Autodesk Inventor part; units mm, degrees
ref_plane "YZ Plane" through (0, 0, 0) normal (1, 0, 0) x (0, 1, 0)
ref_plane "XZ Plane" through (0, 0, 0) normal (0, 1, 0) x (-1, 0, 0)
ref_plane "XY Plane" through (0, 0, 0) normal (0, 0, 1) x (1, 0, 0)
sketch "Skizze1" plane through (0, 0, 0) normal (0, 1, 0) x (-1, 0, 0)
  line L0 (0, 0) -> (-79.5, 0)
  line L1 (-79.5, 0) -> (-79.5, -51.5)
  line L2 (-79.5, -51.5) -> (0, -51.5)
  line L3 (0, -51.5) -> (0, 0)
  line L4 (-30.25, -15.25) -> (-49.25, -15.25)
  line L5 (-49.25, -15.25) -> (-49.25, -36.25)
  line L6 (-49.25, -36.25) -> (-30.25, -36.25)
  line L7 (-30.25, -36.25) -> (-30.25, -15.25)
  point P0 (-39.75, -36.25)
  point P1 (-39.75, -51.5)
  point P2 (-49.25, -25.75)
  point P3 (-79.5, -25.75)
  dimension "d0" = 79.5
  dimension "d1" = 51.5
  dimension "d4" = 21
  dimension "d5" = 19
extrude "Extrusion1" add sketch "Skizze1" along normal blind 3
properties part number "wood_front"
CAD build for the part. Positions are in the model's coordinates, mm. A direction names the side the tool comes from. Round coordinates to 2 decimals unless told otherwise and drop trailing zeros. Order: outer loops, then holes, each group sorted by start corner. A loop starts at its lowest first (then second) coordinate and runs counter-clockwise, first axis right, second up. Notation, with made-up numbers: (34.25, -27.5) -> (53.25, -27.5) arc R19 ccw to (53.25, -9.5) -> close; hole circle Ø2 at (-24, 20.5). An arc over 180 degrees is marked (long way). Write item = value, one per line. Start each with the question number.
(1) Cut at B-B, the plane x = 33. List the corners of the cut face in (y, z), then the cut area to 3 significant figures.
(2) Which spindle directions (+Z, -Z, +X, -X, +Y, -Y) get a long thin tool onto all of the face, cutting with end or side? Do faces 1 (the flat face through (40, 1, -51.5)), 2 (the flat face through (49.25, 1, -26)). Say none if no direction does.
(3) Cut at A-A, the plane z = -35. List the corners of the cut face in (x, y), then the cut area to 4 significant figures.
(4) Cut at C-C, the plane y = 1.3. List the corners of the cut face in (x, z), then the cut area to 3 significant figures.
(5) Probe line 1 (Z direction, x = 41, y = 1.15); line 2 (X direction, y = 0.8, z = -22.5). List the from-to ranges inside material, lowest first. Write a range as [from, to].
(6) Pull direction X, two halves, no side cores. Call faces 3 (the flat face through (79.5, 1, -25)), 4 (the flat face through (40, 0, -14)), 5 (the flat face through (30.25, 1, -26)): released by +X, released by -X, zero draft, split by the parting line, or undercut.
Model answer:
q1.outline = (0, -51.5) -> (3, -51.5) -> (3, -36.25) -> (0, -36.25) -> close; (0, -15.25) -> (3, -15.25) -> (3, 0) -> (0, 0) -> close
q1.area = 91.5 mm2
q2.face_1 = -Z, +X, -X, +Y, -Y
q2.face_2 = +Y, -Y
q3.outline = (0, 0) -> (30.25, 0) -> (30.25, 3) -> (0, 3) -> close; (49.25, 0) -> (79.5, 0) -> (79.5, 3) -> (49.25, 3) -> close
q3.area = 181.5 mm2
q4.outline = (0, -51.5) -> (79.5, -51.5) -> (79.5, 0) -> (0, 0) -> close; hole (30.25, -36.25) -> (49.25, -36.25) -> (49.25, -15.25) -> (30.25, -15.25) -> close
q4.area = 3,700 mm2
q5.line_1 = [-51.5, -36.25], [-15.25, 0]
q5.line_2 = [0, 30.25], [49.25, 79.5]
q6.face_3 = released by +X
q6.face_4 = zero draft
q6.face_5 = undercut
